Source: CAD feature listing. Evaluate the final solid. Frame: model axes, mm. A direction names the side the tool comes from. Coordinates: 2 decimals unless noted, no trailing zeros. Loops run counter-clockwise (first coordinate to the right, second up) from the corner with the lowest first, then second, coordinate; pieces in that order, holes last.
```python
from build123d import *

# Parameters (mm, degrees)
SKETCH2_R                = 1.5
BOSS_EXTRUDE1_DEPTH      = 3
FILLET2_R                = 8
FILLET2_OF_MIRROR1_R     = 8
BOSS_EXTRUDE2_DEPTH      = 55
BOSS_EXTRUDE2_DEPTH_BACK = 55
CUT_EXTRUDE1_REACH       = 134.277
RIB1_REACH               = 202.324
SKETCH6_WALL_W           = 428.260921382
SKETCH6_WALL_H           = 5
FILLET3_R                = 8
CUT_EXTRUDE2_DEPTH       = 165.217203727


with BuildPart() as part:
    # Sketch2 → Boss-Extrude1 (new body)
    with BuildSketch(Plane(origin=(0, -88.5, 0), x_dir=(1, 0, 0), z_dir=(0, 1, 0))):
        with BuildLine():
            Line((-9, -118.2), (-14.150105789, -101.1859937))
            ThreePointArc((-14.150105789, -101.1859937), (-18.012528176, -98.73772981), (-21, -102.2))
            Line((-21, -102.2), (-21, -118.2))
            Line((-21, -118.2), (-55, -130.2))
            Line((-55, -130.2), (-55, -135.2))
            Line((-55, -135.2), (0, -135.2))
            Line((0, -135.2), (0, -118.2))
            Line((0, -118.2), (-9, -118.2))
        make_face()
        with Locations(Location((-17.5, -102.2, 0), (0, 0, 270))):
            Circle(SKETCH2_R, mode=Mode.SUBTRACT)
    boss_extrude1 = extrude(amount=-BOSS_EXTRUDE1_DEPTH)

    # Fillet2
    fillet2_edges = [part.edges().sort_by_distance(p)[0] for p in [
        (-21, -90, 118.2),
        (-9, -90, 118.2),
    ]]
    fillet(fillet2_edges, radius=FILLET2_R)

    # Mirror1: Boss-Extrude1 across plane
    add(boss_extrude1.mirror(Plane(origin=(0, 0, 0), x_dir=(0, 0, 1), z_dir=(1, 0, 0))))

    # Fillet2 of Mirror1
    fillet2_of_mirror1_edges = [part.edges().sort_by_distance(p)[0] for p in [
        (21, -90, 118.2),
        (9, -90, 118.2),
    ]]
    fillet(fillet2_of_mirror1_edges, radius=FILLET2_OF_MIRROR1_R)

    # Sketch4 → Boss-Extrude2 (add, two sides: drawn at the far end of the back side and taken through both)
    with BuildSketch(Plane(origin=(0, 0, 0), x_dir=(0, 0, -1), z_dir=(1, 0, 0)).offset(-BOSS_EXTRUDE2_DEPTH_BACK)):
        Polygon((-135.2, -91.5), (-135.2, -104.5), (-149.7, -104.5), (-149.7, -79.5), (-152.7, -79.5), (-152.7, -107.5), (-132.2, -107.5), (-132.2, -91.5), align=None)
    extrude(amount=BOSS_EXTRUDE2_DEPTH + BOSS_EXTRUDE2_DEPTH_BACK)

    # Sketch5 → Cut-Extrude1 (cut, up to next)
    with BuildSketch(Plane.XY.offset(152.7), mode=Mode.PRIVATE) as cut_extrude1_sk1:
        with BuildLine():
            Line((-35, -93), (-35, -73))
            Line((-35, -73), (-15, -73))
            Line((-15, -73), (-15, -93))
            ThreePointArc((-15, -93), (-25, -103), (-35, -93))
        make_face()
    cut_extrude1_tool1 = extrude(cut_extrude1_sk1.sketch, amount=-CUT_EXTRUDE1_REACH, mode=Mode.PRIVATE) & part.part
    # Sketch5 → Cut-Extrude1 (cut, up to next)
    with BuildSketch(Plane.XY.offset(152.7), mode=Mode.PRIVATE) as cut_extrude1_sk2:
        with BuildLine():
            Line((28, -93), (28, -73))
            Line((28, -73), (48, -73))
            Line((48, -73), (48, -93))
            ThreePointArc((48, -93), (38, -103), (28, -93))
        make_face()
    cut_extrude1_tool2 = extrude(cut_extrude1_sk2.sketch, amount=-CUT_EXTRUDE1_REACH, mode=Mode.PRIVATE) & part.part
    add(cut_extrude1_tool1.solids().sort_by_distance((-25, -87.016415, 152.7))[0], mode=Mode.SUBTRACT)
    add(cut_extrude1_tool2.solids().sort_by_distance((38, -87.016415, 152.7))[0], mode=Mode.SUBTRACT)

    # Sketch6 wall → Rib1 (add, up to next)
    with BuildSketch(Plane(origin=(-17.5, -99.5, 122.2), x_dir=(0, -0.624695047554, 0.780868809443), z_dir=(0, -0.780868809443, -0.624695047554)), mode=Mode.PRIVATE) as rib1_sk1:
        Rectangle(SKETCH6_WALL_W, SKETCH6_WALL_H)
    rib1_tool1 = extrude(rib1_sk1.sketch, amount=-RIB1_REACH, mode=Mode.PRIVATE) - part.part
    rib1 = rib1_tool1.solids().sort_by_distance((-17.5, -99.5, 122.2))[0]
    add(rib1)

    # Mirror2: Rib1 across plane
    add(rib1.mirror(Plane(origin=(0, 0, 0), x_dir=(0, 0, 1), z_dir=(1, 0, 0))))

    # Fillet3
    fillet3_edges = [part.edges().sort_by_distance(p)[0] for p in [
        (-37.5, -91.5, 132.2),
        (37.5, -91.5, 132.2),
        (0, -91.5, 132.2),
    ]]
    fillet(fillet3_edges, radius=FILLET3_R)

    # Sketch7 → Cut-Extrude2 (cut, through all)
    with BuildSketch(Plane(origin=(0, -104.5, 0), x_dir=(1, 0, 0), z_dir=(0, 1, 0))):
        with BuildLine():
            Line((-30, -140.45), (25.5, -140.45))
            ThreePointArc((25.5, -140.45), (26.7, -141.65), (25.5, -142.85))
            Line((25.5, -142.85), (-30, -142.85))
            ThreePointArc((-30, -142.85), (-31.2, -141.65), (-30, -140.45))
        make_face()
    extrude(amount=-CUT_EXTRUDE2_DEPTH, mode=Mode.SUBTRACT)


solid = part.part
```
Q1. Material intervals for line 1 along X through (y, z) = (-82.5, 150); line 2 along Z through (x, y) = (17.5, -90.75); line 3 along X through (y, z) = (-89.5, 102.2), sorted ascending.
Q2. Section query D-D on y = -97.5. Return the cut outline in (x, z).
Q3. Section query C-C on z = 141.65. Return the cut outline in (x, y), then the cut area to 3 significant figures.
Q4. Section query B-B on x = 17.5. Return the cut outline in (y, z), then the cut area to 3 significant figures.
Q5. First-contact query: pin 1 Ø9 at (x, y) = (3.5, -103.5) entering from -Z; pin 2 Ø2.5 at (y, z) = (-90.5, 106.5) entering from -X; pin 3 Ø7.5 at (x, y) = (12, -91.5) entering from -Z. Flat tips, straight axial feed; report the tip coordinate or a pass-through.
Q6. Section query A-A on y = -86.5. Return the cut outline in (x, z), then the cut area to 3 significant figures.
Q7. Draft query along X for faces 5 (the cylindrical face through (0.21, -93.781, 129.794)), 6 (the flat face through (-1, -96, 135.2)), 7 (the flat face through (20, -97, 124)). Return one class per face: released by +X, released by -X, zero draft, split by the parting line, or undercut.
Q8. Reachability of faces 1 (the flat face through (-1, -92, 149.7)), 2 (the cylindrical face through (38, -103, 151)), 3 (the cylindrical face through (37.745, -93.781, 129.794)), 4 (the flat face through (-2, -106, 142.85)) from +Z, -Z, +X, -X, +Y, -Y: full face, straight path, thin tool, end or side. Return the list, or none.
Resolved:
1. line 1: x = -55 to -35, -15 to 28, 48 to 55
1. line 2: z = 98.7 to 100.7, 103.7 to 135.2, 149.7 to 152.7
1. line 3: x = -21 to -19, -16 to -13.84, 13.84 to 16, 19 to 21
2. outline: (-55, 131.95) - (-20, 131.95) - (-20, 119.7) - (-15, 119.7) - (-15, 131.95) - (15, 131.95) - (15, 119.7) - (20, 119.7) - (20, 131.95) - (55, 131.95) - (55, 135.2) - (-55, 135.2) - close; (-55, 149.7) - (-33.93, 149.7) - (-33.93, 152.7) - (-55, 152.7) - close; (-16.07, 149.7) - (29.07, 149.7) - (29.07, 152.7) - (-16.07, 152.7) - close; (46.93, 149.7) - (55, 149.7) - (55, 152.7) - (46.93, 152.7) - close
3. outline: (-55, -107.5) - (-31.2, -107.5) - (-31.2, -104.5) - (-55, -104.5) - close; (26.7, -107.5) - (55, -107.5) - (55, -104.5) - (26.7, -104.5) - close
3. area: 156 mm2
4. outline: (-107.5, 132.2) - (-91.5, 112.2) - (-91.5, 103.7) - (-88.5, 103.7) - (-88.5, 135.2) - (-104.5, 135.2) - (-104.5, 140.45) - (-107.5, 140.45) - close; (-107.5, 142.85) - (-104.5, 142.85) - (-104.5, 149.7) - (-79.5, 149.7) - (-79.5, 152.7) - (-107.5, 152.7) - close; (-91.5, 98.7) - (-88.5, 98.7) - (-88.5, 100.7) - (-91.5, 100.7) - close
4. area: 429 mm2
5. pin 1: stops at z = 132.18
5. pin 2: stops at x = -21
5. pin 3: stops at z = 99.17
6. outline: (-55, 149.7) - (-35, 149.7) - (-35, 152.7) - (-55, 152.7) - close; (-15, 149.7) - (28, 149.7) - (28, 152.7) - (-15, 152.7) - close; (48, 149.7) - (55, 149.7) - (55, 152.7) - (48, 152.7) - close
6. area: 210 mm2
7. face 5: undercut
7. face 6: zero draft
7. face 7: released by +X
8. face 1: +X, -X, +Y
8. face 2: +Z, +Y
8. face 3: -Z, +X, -Y
8. face 4: +Y, -Y
